Input: part model. Units: mm. Frame: model coordinates. Face numbers are marked on the shaded views. Coordinates: 2 decimals unless noted, no trailing zeros. Write each loop counter-clockwise with the first axis right and the second up, starting at its lowest first coordinate (ties: lowest second). Pieces come first, ordered by that corner, then holes.
1) Pin query (flat end, axial travel): pin 1 Ø1 at (x, z) = (-27.5, 57.5) entering from +Y; pin 2 Ø7 at (x, y) = (-7, 7.5) entering from +Z. Return the tip coordinate at first contact, or that it passes through.
2) Section query A-A (z = 18). Output: boundary loops of the cut face in (x, y), then the cut area to 3 significant figures.
3) Section query B-B (x = 4). Output: boundary loops of the cut face in (y, z), then the cut area to 3 significant figures.
4) Line query: L1, parallel to X at y = 11, z = 37; L2, parallel to Z at x = -3.5, y = 10; L3, parallel to Y at x = -21.5, z = 10. Output: solid intervals per line, ascending.
5) Section query C-C (y = 9.25). Output: boundary loops of the cut face in (x, z).
6) Draft query along X for the marked faces 1, 2 and 3. Return one class per face: pulls with the +X half, pulls with the -X half, needs draft (parallel to the pull), parting line crosses it, or undercut.
from build123d import *

# Parameters (mm, degrees)
F1_DEPTH = 70
F3_DEPTH = 3
F4_R     = 2
F5_R     = 1


with BuildPart() as f1:
    # F0 (on Top) → F1 (new body)
    with BuildSketch(Plane.XY):
        Polygon((-41.2, 0), (0, 0), (0, 2.2), (-39, 2.2), (-39, 13.7), (-35, 13.7), (-35, 15.9), (-41.2, 15.9), align=None)
        Polygon((0, 2.2), (0, 0), (41.2, 0), (41.2, 14.6), (41.2, 15.9), (35, 15.9), (35, 13.7), (39, 13.7), (39, 2.2), align=None)
    extrude(amount=F1_DEPTH)

    # F2 (on face) → F3 (join)
    with BuildSketch(Plane.XY):
        Polygon((0, 0), (41.2, 0), (41.2, 15.9), (-35, 15.9), (-35, 13.7), (-39, 13.7), (-39, 2.2), (0, 2.2), align=None)
        Polygon((-41.2, 0), (0, 0), (0, 2.2), (-39, 2.2), (-39, 13.7), (-35, 13.7), (-35, 15.9), (-41.2, 15.9), align=None)
    extrude(amount=F3_DEPTH)

    # F4
    f4_edges = [f1.edges().sort_by_distance(p)[0] for p in [
        (41.2, 0, 35),
        (41.2, 15.9, 35),
        (35, 15.9, 36.5),
        (39, 2.2, 36.5),
        (-35, 15.9, 36.5),
        (-39, 2.2, 36.5),
        (-41.2, 15.9, 35),
        (-41.2, 0, 35),
        (0, 0, 0),
        (0, 15.9, 0),
        (-41.2, 7.95, 0),
        (41.2, 7.95, 0),
    ]]
    fillet(f4_edges, radius=F4_R)

    # F5
    f5_edges = [f1.edges().sort_by_distance(p)[0] for p in [
        (0, 2.2, 70),
        (0, 0, 70),
    ]]
    fillet(f5_edges, radius=F5_R)


solid = f1.part
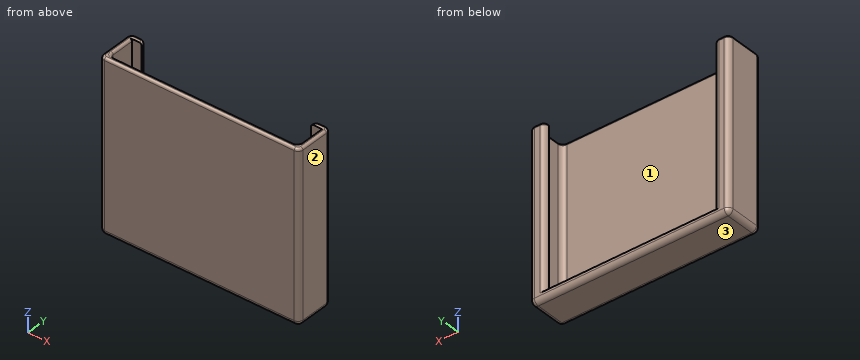
Answer:
1. pin 1: stops at y = 2.2
1. pin 2: stops at z = 3
2. outline: (-41.2, 2) arc R2 ccw to (-39.2, 0) - (39.2, 0) arc R2 ccw to (41.2, 2) - (41.2, 13.9) arc R2 ccw to (39.2, 15.9) - (37, 15.9) arc R2 ccw to (35, 13.9) - (35, 13.7) - (39, 13.7) - (39, 4.2) arc R2 cw to (37, 2.2) - (-37, 2.2) arc R2 cw to (-39, 4.2) - (-39, 13.7) - (-35, 13.7) - (-35, 13.9) arc R2 ccw to (-37, 15.9) - (-39.2, 15.9) arc R2 ccw to (-41.2, 13.9) - close
2. area: 256 mm2
3. outline: (0, 2) arc R2 ccw to (2, 0) - (13.9, 0) arc R2 ccw to (15.9, 2) - (15.9, 3) - (2.2, 3) - (2.2, 69) arc R1 ccw to (1.2, 70) - (1, 70) arc R1 ccw to (0, 69) - close
3. area: 193 mm2
4. L1: x = -41.2 to -39, 39 to 41.2
4. L2: z = 0 to 3
4. L3: y = 0 to 2.2
5. outline: (-41.2, 2) arc R2 ccw to (-39.2, 0) - (39.2, 0) arc R2 ccw to (41.2, 2) - (41.2, 69) arc R1 ccw to (40.2, 70) - (40, 70) arc R1 ccw to (39, 69) - (39, 3) - (-39, 3) - (-39, 69) arc R1 ccw to (-40, 70) - (-40.2, 70) arc R1 ccw to (-41.2, 69) - close
6. face 1: undercut
6. face 2: pulls with the +X half
6. face 3: needs draft
